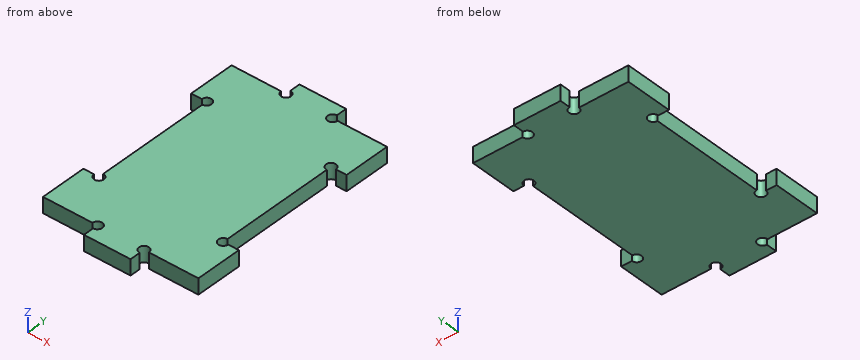
from build123d import *

# Parameters (mm, degrees)
BOSS_EXTRUDE2_DEPTH = 5
SKETCH3_W           = 5
SKETCH3_H           = 40
CUT_EXTRUDE1_DEPTH  = 5
SKETCH4_R           = 1.5875
CUT_EXTRUDE2_DEPTH  = 6


with BuildPart() as part:
    # Sketch2 → Boss-Extrude2 (new body)
    with BuildSketch(Plane.XY):
        Polygon((-7.5, 40), (7.5, 40), (7.5, 35), (25, 35), (25, -35), (7.5, -35), (7.5, -40), (-7.5, -40), (-7.5, -35), (-25, -35), (-25, 35), (-7.5, 35), align=None)
    extrude(amount=BOSS_EXTRUDE2_DEPTH)

    # Sketch3 → Cut-Extrude1 (cut)
    with BuildSketch(Plane.XY.offset(5)):
        with Locations((-22.5, 0)):
            Rectangle(SKETCH3_W, SKETCH3_H)
    cut_extrude1 = extrude(amount=-CUT_EXTRUDE1_DEPTH, mode=Mode.SUBTRACT)

    # Mirror1: Cut-Extrude1 across plane
    add(cut_extrude1.mirror(Plane(origin=(0, 0, 0), x_dir=(0, 0, 1), z_dir=(1, 0, 0))), mode=Mode.SUBTRACT)

    # Sketch4 → Cut-Extrude2 (cut, through all)
    with BuildSketch(Plane.XY.offset(5)):
        with Locations((-7.5, 35)):
            Circle(SKETCH4_R)
        with Locations((7.5, 35)):
            Circle(SKETCH4_R)
        with Locations((20, 20)):
            Circle(SKETCH4_R)
        with Locations((-20, 20)):
            Circle(SKETCH4_R)
        with Locations((-20, -20)):
            Circle(SKETCH4_R)
        with Locations((-7.5, -35)):
            Circle(SKETCH4_R)
        with Locations((7.5, -35)):
            Circle(SKETCH4_R)
        with Locations((20, -20)):
            Circle(SKETCH4_R)
    extrude(amount=-CUT_EXTRUDE2_DEPTH, mode=Mode.SUBTRACT)


solid = part.part
Model file for the job. Use its own axes, mm. Give positions to 0.01 mm unless a question says otherwise; leave off trailing zeros. Write each loop counter-clockwise with the first axis right and the second up, starting at its lowest first coordinate (ties: lowest second). Pieces come first, ordered by that corner, then holes. Notation, with made-up numbers: M -18.75,-21.75 L -9.75,-21.75 A29 ccw -9.75,0.25 Z; hole C 57,-8 d9. An arc over 180 degrees is marked long. One line per item, written item: value. Start each with the question number.
Q1. Saw through at A-A, the plane z = 3.65. Write the cut outline in (x, y) (1 decimal), plus the area to 3 significant figures.
Q2. Drop flat-ended pins along their axis: pin 1 Ø1.5 at (x, z) = (-20.5, 2.5) entering from +Y; pin 2 Ø2.5 at (y, z) = (-9, 2.5) entering from +X; pin 3 Ø1 at (y, z) = (-38, 2) entering from +X; pin 4 Ø4 at (x, y) = (-4.5, 20) entering from -Z. Give the stop position or say it passes through.
Q3. Probe probe 1 along Y at (x, z) = (-7, 4.6); probe 2 along Y at (x, z) = (-19, 2.55); probe 3 along X at (y, z) = (1.5, 1.65). List the from-to ranges inside material, lowest first. Write a range as [from, to].
Q4. Saw through at B-B, the plane y = 10. Write the cut outline in (x, z).
Output values:
1. outline: M -25,-35 L -9.1,-35 A1.6 cw long -7.5,-36.6 L -7.5,-40 L 7.5,-40 L 7.5,-36.6 A1.6 cw long 9.1,-35 L 25,-35 L 25,-20 L 21.6,-20 A1.6 cw long 20,-18.4 L 20,18.4 A1.6 cw long 21.6,20 L 25,20 L 25,35 L 9.1,35 A1.6 cw long 7.5,36.6 L 7.5,40 L -7.5,40 L -7.5,36.6 A1.6 cw long -9.1,35 L -25,35 L -25,20 L -21.6,20 A1.6 cw long -20,18.4 L -20,-18.4 A1.6 cw long -21.6,-20 L -25,-20 Z
1. area: 3,200 mm²
2. pin 1: stops at y = 35
2. pin 2: stops at x = 20
2. pin 3: stops at x = 7.5
2. pin 4: stops at z = 0
3. probe 1: y = [-40, -36.51], [-33.49, 33.49], [36.51, 40]
3. probe 2: y = [-35, -21.23], [-18.77, 18.77], [21.23, 35]
3. probe 3: x = [-20, 20]
4. outline: M -20,0 L 20,0 L 20,5 L -20,5 Z
